Can you work these out from the model? Positions are in its coordinate system, mm. A direction names the side the tool comes from. Round coordinates to 2 decimals unless told otherwise and drop trailing zeros. Write each loop counter-clockwise with the first axis right and the second up, starting at its lowest first coordinate (ties: lowest second). Pieces come first, ordered by that corner, then holes. Notation, with made-up numbers: M 11,45 L 16,45 A22 cw 16,70 Z; hole C 78,62 d2. An arc over 180 degrees is marked long. Use one line per item in the form item = value. Start each with the question number.
```python
from build123d import *

# Parameters (mm, degrees)
EXTRUDE_1_DEPTH = 30


with BuildPart() as part:
    # 草图1 → 凸台-拉伸1 (new body)
    with BuildSketch(Plane.XY):
        with BuildLine():
            Line((-28.427104886, 7.685760518), (-20.027104886, 7.685760518))
            ThreePointArc((-20.027104886, 7.685760518), (-19.814972852, 7.773628483), (-19.727104886, 7.985760518))
            Line((-19.727104886, 7.985760518), (-19.727104886, 13.385760518))
            ThreePointArc((-19.727104886, 13.385760518), (-19.814972852, 13.597892552), (-20.027104886, 13.685760518))
            Line((-20.027104886, 13.685760518), (-22.177104886, 13.685760518))
            ThreePointArc((-22.177104886, 13.685760518), (-22.389236921, 13.597892552), (-22.477104886, 13.385760518))
            Line((-22.477104886, 13.385760518), (-22.477104886, 12.435760518))
            ThreePointArc((-22.477104886, 12.435760518), (-22.389236921, 12.223628483), (-22.177104886, 12.135760518))
            Line((-22.177104886, 12.135760518), (-21.277104886, 12.135760518))
            Line((-21.277104886, 12.135760518), (-21.277104886, 9.235760518))
            Line((-21.277104886, 9.235760518), (-27.177104886, 9.235760518))
            Line((-27.177104886, 9.235760518), (-27.177104886, 12.135760518))
            Line((-27.177104886, 12.135760518), (-26.277104886, 12.135760518))
            ThreePointArc((-26.277104886, 12.135760518), (-26.064972852, 12.223628483), (-25.977104886, 12.435760518))
            Line((-25.977104886, 12.435760518), (-25.977104886, 13.385760518))
            ThreePointArc((-25.977104886, 13.385760518), (-26.064972852, 13.597892552), (-26.277104886, 13.685760518))
            Line((-26.277104886, 13.685760518), (-28.427104886, 13.685760518))
            ThreePointArc((-28.427104886, 13.685760518), (-28.639236921, 13.597892552), (-28.727104886, 13.385760518))
            Line((-28.727104886, 13.385760518), (-28.727104886, 7.985760518))
            ThreePointArc((-28.727104886, 7.985760518), (-28.639236921, 7.773628483), (-28.427104886, 7.685760518))
        make_face()
    extrude(amount=EXTRUDE_1_DEPTH)


solid = part.part
```
1. If we section it at C-C (y = 11.5): List the corners of the cut face in (x, z) for me, and give its area (3 significant figures).
2. If we section it at D-D (x = -24.75): List the corners of the cut face in (y, z) for me.
3. If we section it at A-A (y = 12.75): List the corners of the cut face in (x, z) for me, and give its area (3 significant figures).
4. If we mould it in two halves opening along Y, with no side actions, what happens to faces 1 (the face through (-27, 13.686, 15)), 2 (the face through (-24, 7.686, 15)), 3 (the face through (-22, 12.136, 15))? For each: pulls with the +Y half, pulls with the -Y half, needs draft (parallel to the pull), parting line crosses it, or undercut.
5. Please list where these lines run through material, in increasing order: line 1 along Y through (x, z) = (-27, 22); line 2 along X through (y, z) = (9.75, 4); line 3 along X through (y, z) = (13, 27.75).
6. If we section it at B-B (z = 8): List the corners of the cut face in (x, y) for me, and give its area (3 significant figures).
7. Which directions (+Z, -Z, +X, -X, +Y, -Y) give clear straight access to the entire face, cutting with the end or side of a thin tool? Please do faces 4 (the face through (-22.477, 13, 15)), 5 (the face through (-24, 9, 30)), 6 (the face through (-24, 9.236, 15)).
Model answer:
q1.outline = M -28.73,0 L -27.18,0 L -27.18,30 L -28.73,30 Z; M -21.28,0 L -19.73,0 L -19.73,30 L -21.28,30 Z
q1.area = 93.0 mm2
q2.outline = M 7.69,0 L 9.24,0 L 9.24,30 L 7.69,30 Z
q3.outline = M -28.73,0 L -25.98,0 L -25.98,30 L -28.73,30 Z; M -22.48,0 L -19.73,0 L -19.73,30 L -22.48,30 Z
q3.area = 165 mm2
q4.face_1 = pulls with the +Y half
q4.face_2 = pulls with the -Y half
q4.face_3 = undercut
q5.line_1 = 7.69 to 9.24, 12.14 to 13.69
q5.line_2 = -28.73 to -27.18, -21.28 to -19.73
q5.line_3 = -28.73 to -25.98, -22.48 to -19.73
q6.outline = M -28.73,7.99 A0.3 ccw -28.43,7.69 L -20.03,7.69 A0.3 ccw -19.73,7.99 L -19.73,13.39 A0.3 ccw -20.03,13.69 L -22.18,13.69 A0.3 ccw -22.48,13.39 L -22.48,12.44 A0.3 ccw -22.18,12.14 L -21.28,12.14 L -21.28,9.24 L -27.18,9.24 L -27.18,12.14 L -26.28,12.14 A0.3 ccw -25.98,12.44 L -25.98,13.39 A0.3 ccw -26.28,13.69 L -28.43,13.69 A0.3 ccw -28.73,13.39 Z
q6.area = 31.3 mm2
q7.face_4 = +Z, -Z, +Y
q7.face_5 = +Z, +X, -X, +Y, -Y
q7.face_6 = +Z, -Z
